Model file for the job. Use its own axes, mm. A direction names the side the tool comes from. Round coordinates to 2 decimals unless told otherwise and drop trailing zeros. Write each loop counter-clockwise with the first axis right and the second up, starting at its lowest first coordinate (ties: lowest second). Pieces come first, ordered by that corner, then holes. Notation, with made-up numbers: (-7.75, 89) - (42.25, 89) arc R9 ccw to (42.25, 100) - close; hole circle Ø6 at (-23.75, 42). An arc over 180 degrees is marked (long way). One line per item, written item: value.
Autodesk Inventor part; units mm, degrees
ref_plane "YZ Plane" through (0, 0, 0) normal (1, 0, 0) x (0, 1, 0)
ref_plane "XZ Plane" through (0, 0, 0) normal (0, 1, 0) x (-1, 0, 0)
ref_plane "XY Plane" through (0, 0, 0) normal (0, 0, 1) x (1, 0, 0)
sketch "Sketch1" plane through (0, 0, 0) normal (0, 0, 1) x (1, 0, 0)
  line L0 (-43.5443, 19.427) -> (49.4557, 19.427)
  line L1 (52.4557, 16.427) -> (52.4557, -43.573)
  line L2 (49.4557, -46.573) -> (-43.5443, -46.573)
  line L3 (-46.5443, -43.573) -> (-46.5443, 16.427)
  arc A0 (-43.5443, 19.427) -> (-46.5443, 16.427) centre (-43.5443, 16.427) ccw
  arc A1 (-46.5443, -43.573) -> (-43.5443, -46.573) centre (-43.5443, -43.573) ccw
  arc A2 (49.4557, -46.573) -> (52.4557, -43.573) centre (49.4557, -43.573) ccw
  arc A3 (52.4557, 16.427) -> (49.4557, 19.427) centre (49.4557, 16.427) ccw
  point P0 (0, 0)
  point P1 (0, 0)
  point P2 (-46.5443, 19.427)
  point P3 (52.4557, -46.573)
  point P4 (52.4557, 19.427)
  dimension "d0" = 99
  dimension "d1" = 66
  dimension "d2" = 3
extrude "Extrusion1" add sketch "Sketch1" along normal blind 1.27
sketch "Sketch2" plane through (0, 0, 1.27) normal (0, 0, 1) x (1, 0, 0)
  line L0 (-46.5443, 16.427) -> (-46.5443, -43.573)
  line L1 (49.4557, 19.427) -> (-43.5443, 19.427)
  circle A0 centre (-42.7343, 15.617) radius 1.5875
  line L2 (-50.0562, -13.573) -> (79.0191, -13.573) construction
  line L3 (2.9557, 30.2203) -> (2.9557, -48.7988) construction
  circle A1 centre (-42.7343, -42.763) radius 1.5875
  circle A2 centre (48.6457, 15.617) radius 1.5875
  circle A3 centre (48.6457, -42.763) radius 1.5875
  point P0 (0, 0)
  dimension "d8" = 3.175
  dimension "d9" = 3.81
  dimension "d10" = 3.81
extrude "Extrusion2" cut sketch "Sketch2" against normal blind 25.4
sketch "Sketch3" plane through (0, 0, 1.27) normal (0, 0, 1) x (1, 0, 0)
  circle A0 centre (48.6457, 15.617) radius 1.5875
  circle A1 centre (-42.7343, 15.617) radius 1.5875
  circle A2 centre (-42.7343, -42.763) radius 1.5875
  circle A3 centre (48.6457, -42.763) radius 1.5875
  line L0 (49.4557, 19.427) -> (-43.5443, 19.427)
  arc A4 (-43.5443, 19.427) -> (-46.5443, 16.427) centre (-43.5443, 16.427) ccw
  line L1 (-46.5443, 16.427) -> (-46.5443, -43.573) construction
  arc A5 (-46.5443, -43.573) -> (-43.5443, -46.573) centre (-43.5443, -43.573) ccw
  line L2 (-43.5443, -46.573) -> (49.4557, -46.573)
  arc A6 (49.4557, -46.573) -> (52.4557, -43.573) centre (49.4557, -43.573) ccw
  line L3 (52.4557, -43.573) -> (52.4557, 16.427)
  arc A7 (52.4557, 16.427) -> (49.4557, 19.427) centre (49.4557, 16.427) ccw
  arc A8 (-43.5443, 19.427) -> (-46.5443, 16.427) centre (-43.5443, 16.427) ccw
  line L4 (49.4557, 19.427) -> (-43.5443, 19.427)
  circle A9 centre (48.6457, 15.617) radius 1.5875
  circle A10 centre (-42.7343, 15.617) radius 1.5875
  circle A11 centre (-42.7343, -42.763) radius 1.5875
  circle A12 centre (48.6457, -42.763) radius 1.5875
  arc A13 (52.4557, 16.427) -> (49.4557, 19.427) centre (49.4557, 16.427) ccw
  line L5 (52.4557, 16.427) -> (52.4557, -43.573)
  arc A14 (49.4557, -46.573) -> (52.4557, -43.573) centre (49.4557, -43.573) ccw
  line L6 (49.4557, -46.573) -> (-43.5443, -46.573)
  arc A15 (-46.5443, -43.573) -> (-43.5443, -46.573) centre (-43.5443, -43.573) ccw
  line L7 (-46.5443, -43.573) -> (-46.5443, 16.427)
  arc A16 (-43.5443, 19.427) -> (-46.5443, 16.427) centre (-43.5443, 16.427) ccw
  line L8 (-43.5443, 19.427) -> (49.4557, 19.427)
  line L9 (-43.5443, 19.427) -> (49.4557, 19.427)
  line L10 (-40.8039, 19.427) -> (-40.8039, -46.573) construction
  line L11 (49.4557, -46.573) -> (-43.5443, -46.573)
  line L12 (-40.8039, 19.427) -> (-51.3078, 19.427) construction
  line L13 (-40.8039, -46.573) -> (-51.3078, -46.573) construction
  line L14 (-40.8039, -21.173) -> (-51.3078, -21.173) construction
  line L15 (-40.8039, -5.973) -> (-51.3078, -5.973) construction
  line L16 (-46.5443, -43.573) -> (-46.5443, 16.427)
  line L17 (-46.5443, -5.973) -> (-40.8039, -5.973)
  line L18 (-40.8039, -5.973) -> (-40.8039, -21.173)
  line L19 (-40.8039, -21.173) -> (-46.5443, -21.173)
  line L20 (-46.5443, -21.173) -> (-46.5443, -5.973)
  point P0 (0, 0)
  dimension "d13" = 25.4
  dimension "d14" = 25.4
  dimension "d15" = 5.7404
extrude "Extrusion3" cut sketch "Sketch3" against normal blind 25.4 contours L17 L18 L19 L7
fillet "Fillet1" radius 3.175 2 edges at (-46.5443, -21.173, 0.635) (-46.5443, -5.973, 0.635)
sketch "Sketch9" plane through (0, 0, 1.27) normal (0, 0, 1) x (1, 0, 0)
  arc A0 (-43.5443, 19.427) -> (-46.5443, 16.427) centre (-43.5443, 16.427) ccw
  line L0 (-46.5443, -2.798) -> (-46.5443, 16.427) construction
  line L1 (-46.5443, 16.427) -> (-46.5443, -2.798)
  line L2 (-43.5443, 19.427) -> (-26.5771, 19.427) construction
  line L3 (49.4557, 19.427) -> (-43.5443, 19.427)
  line L4 (-45.6657, 18.5483) -> (-26.5771, -0.5403) construction
  line L5 (-45.6657, 18.5483) -> (-18.6704, 18.5483) construction
  circle A1 centre (-45.6657, 18.5483) radius 7.1603
  arc A2 (-46.5443, -2.798) -> (-43.3693, -5.973) centre (-43.3693, -2.798) ccw
  line L6 (-43.3693, -5.973) -> (-40.8039, -5.973)
  line L7 (-40.8039, -5.973) -> (-40.8039, -21.173)
  line L8 (-40.8039, -21.173) -> (-43.3693, -21.173)
  arc A3 (-43.3693, -21.173) -> (-46.5443, -24.348) centre (-43.3693, -24.348) ccw
  line L9 (-46.5443, -24.348) -> (-46.5443, -43.573)
  arc A4 (-46.5443, -43.573) -> (-43.5443, -46.573) centre (-43.5443, -43.573) ccw
  line L10 (-43.5443, -46.573) -> (49.4557, -46.573)
  arc A5 (49.4557, -46.573) -> (52.4557, -43.573) centre (49.4557, -43.573) ccw
  line L11 (52.4557, -43.573) -> (52.4557, 16.427)
  arc A6 (52.4557, 16.427) -> (49.4557, 19.427) centre (49.4557, 16.427) ccw
  line L12 (49.4557, 19.427) -> (-43.5443, 19.427)
  arc A7 (-43.5443, 19.427) -> (-46.5443, 16.427) centre (-43.5443, 16.427) ccw
  line L13 (-46.5443, 16.427) -> (-46.5443, -2.798)
  circle A8 centre (48.6457, 15.617) radius 1.5875
  circle A9 centre (-42.7343, 15.617) radius 1.5875
  circle A10 centre (-42.7343, -42.763) radius 1.5875
  circle A11 centre (48.6457, -42.763) radius 1.5875
  line L14 (-75.7777, -13.573) -> (114.1059, -13.573) construction
  line L15 (2.9557, 31.1348) -> (2.9557, -53.319) construction
  circle A12 centre (-45.6657, -45.6944) radius 7.1603
  line L16 (2.9557, -58.2809) -> (2.9557, 26.1729) construction
  circle A13 centre (51.577, 18.5483) radius 7.1603
  circle A14 centre (51.577, -45.6944) radius 7.1603
  point P0 (0, 0)
  dimension "d28" = 45
extrude "Extrusion5" cut sketch "Sketch9" against normal blind 12.7 contours L3 A1 L1 A0 | A0 L1 A1 L3 | A13 L11 A6 L3 | L3 A6 L11 A13 | A14 L10 A5 L11 | L11 A5 L10 A14 | A12 L9 A4 L10 | L10 A4 L9 A12
sketch "Sketch10" plane through (0, 0, 1.27) normal (0, 0, 1) x (1, 0, 0)
  arc A0 (52.4557, -38.5882) -> (44.4708, -46.573) centre (51.577, -45.6944) ccw
  line L0 (52.4557, -38.5882) -> (52.4557, 11.4421)
  arc A1 (44.4708, 19.427) -> (52.4557, 11.4421) centre (51.577, 18.5483) ccw
  line L1 (44.4708, 19.427) -> (-38.5595, 19.427)
  arc A2 (-46.5443, 11.4421) -> (-38.5595, 19.427) centre (-45.6657, 18.5483) ccw
  line L2 (-46.5443, 11.4421) -> (-46.5443, -2.798)
  arc A3 (-46.5443, -2.798) -> (-43.3693, -5.973) centre (-43.3693, -2.798) ccw
  line L3 (-43.3693, -5.973) -> (-40.8039, -5.973)
  line L4 (-40.8039, -5.973) -> (-40.8039, -21.173)
  line L5 (-40.8039, -21.173) -> (-43.3693, -21.173)
  arc A4 (-43.3693, -21.173) -> (-46.5443, -24.348) centre (-43.3693, -24.348) ccw
  line L6 (-46.5443, -24.348) -> (-46.5443, -38.5882)
  arc A5 (-38.5595, -46.573) -> (-46.5443, -38.5882) centre (-45.6657, -45.6944) ccw
  line L7 (-38.5595, -46.573) -> (44.4708, -46.573)
  line L8 (-36.7645, -45.303) -> (43.1467, -45.303)
  line L9 (-36.7645, 18.157) -> (43.1467, 18.157)
  line L10 (44.4708, 19.427) -> (-38.5595, 19.427)
  line L11 (-36.7645, -45.303) -> (-37.2353, -45.303)
  arc A6 (-38.5595, -46.573) -> (-46.5443, -38.5882) centre (-45.6657, -45.6944) ccw
  line L12 (-36.7645, 18.157) -> (-37.2353, 18.157)
  line L13 (51.1857, 10.118) -> (51.1857, -37.264)
  arc A7 (44.4708, 19.427) -> (52.4557, 11.4421) centre (51.577, 18.5483) ccw
  line L14 (-39.5339, -5.973) -> (-39.5339, -21.173)
  line L15 (-45.2743, -2.798) -> (-39.5339, -5.973)
  line L16 (-39.5339, -21.173) -> (-45.2743, -24.348)
  line L17 (51.1857, 10.118) -> (52.4557, 10.118) construction
  line L18 (52.4557, -38.5882) -> (52.4557, 11.4421)
  line L19 (43.1467, 18.157) -> (43.1467, 19.427) construction
  arc A8 (43.1467, 18.157) -> (51.1857, 10.118) centre (51.577, 18.5483) ccw
  line L20 (-56.5649, -13.573) -> (80.9191, -13.573) construction
  line L21 (2.9557, 34.2968) -> (2.9557, -68.6615) construction
  arc A9 (51.1857, -37.264) -> (43.1467, -45.303) centre (51.577, -45.6944) ccw
  arc A10 (-45.2743, 10.118) -> (-37.2353, 18.157) centre (-45.6657, 18.5483) ccw
  arc A11 (-37.2353, -45.303) -> (-45.2743, -37.264) centre (-45.6657, -45.6944) ccw
  line L22 (-45.2743, 10.118) -> (-45.2743, -2.798)
  line L23 (-45.2743, -37.264) -> (-45.2743, -24.348)
  line L24 (-46.5443, -43.573) -> (-46.5443, -24.348)
  point P0 (0, 0)
  dimension "d31" = 1.27
  dimension "d32" = 1.27
  dimension "d35" = 1.27
  dimension "d36" = 1.27
  dimension "d39" = 3.175
  dimension "d40" = 3.175
  dimension "d42" = 1.27
  dimension "d43" = 1.27
  dimension "d44" = 1.2791
extrude "Extrusion6" cut sketch "Sketch10" against normal blind 7.62 contours L11 A11 L23 L16 L14 L15 L22 A10 L12 L9 A8 L13 A9 L8
sketch "Sketch13" plane through (0, 0, 1.27) normal (0, 0, 1) x (1, 0, 0)
  arc A0 (51.1857, -37.264) -> (43.1467, -45.303) centre (51.577, -45.6944) ccw
  line L0 (43.1467, -45.303) -> (-37.2353, -45.303)
  arc A1 (-37.2353, -45.303) -> (-45.2743, -37.264) centre (-45.6657, -45.6944) ccw
  line L1 (-45.2743, -37.264) -> (-45.2743, -24.348)
  line L2 (-45.2743, -24.348) -> (-39.5339, -21.173)
  line L3 (-39.5339, -21.173) -> (-39.5339, -5.973)
  line L4 (-39.5339, -5.973) -> (-45.2743, -2.798)
  line L5 (-45.2743, -2.798) -> (-45.2743, 10.118)
  arc A2 (-45.2743, 10.118) -> (-37.2353, 18.157) centre (-45.6657, 18.5483) ccw
  line L6 (-37.2353, 18.157) -> (43.1467, 18.157)
  arc A3 (43.1467, 18.157) -> (51.1857, 10.118) centre (51.577, 18.5483) ccw
  line L7 (51.1857, 10.118) -> (51.1857, -37.264)
  arc A4 (52.4557, -38.5882) -> (44.4708, -46.573) centre (51.577, -45.6944) ccw
  line L8 (52.4557, -38.5882) -> (52.4557, 11.4421)
  arc A5 (44.4708, 19.427) -> (52.4557, 11.4421) centre (51.577, 18.5483) ccw
  line L9 (44.4708, 19.427) -> (-38.5595, 19.427)
  arc A6 (-46.5443, 11.4421) -> (-38.5595, 19.427) centre (-45.6657, 18.5483) ccw
  line L10 (-46.5443, 11.4421) -> (-46.5443, -2.798)
  arc A7 (-46.5443, -2.798) -> (-43.3693, -5.973) centre (-43.3693, -2.798) ccw
  line L11 (-43.3693, -5.973) -> (-40.8039, -5.973)
  line L12 (-40.8039, -5.973) -> (-40.8039, -21.173)
  line L13 (-40.8039, -21.173) -> (-43.3693, -21.173)
  arc A8 (-43.3693, -21.173) -> (-46.5443, -24.348) centre (-43.3693, -24.348) ccw
  line L14 (-46.5443, -24.348) -> (-46.5443, -38.5882)
  arc A9 (-38.5595, -46.573) -> (-46.5443, -38.5882) centre (-45.6657, -45.6944) ccw
  line L15 (-38.5595, -46.573) -> (44.4708, -46.573)
  point P0 (0, 0)
extrude "Extrusion9" add sketch "Sketch13" along normal blind 1.27 and the other way blind 1.27 contours A0 L0 A1 L1 L2 L3 L4 L5 A2 L6 A3 L7
properties part number "battbase__lid_final"
1. Tool access for faces 4 (the face through (-45.64, -22.13, 0.63)), 5 (the face through (45.548, -39.789, 1.896)), 6 (the face through (-42.36, -4.41, 1.9)): list every direction of +Z, -Z, +X, -X, +Y, -Y with a clear straight run to the whole face (end or side of a thin tool).
Report:
face 4: +Z, -Z, -X
face 5: +Z, +X, -Y
face 6: +Z, -X
2. Band-saw the part on A-A on y = -19.5. Write the cut outline in (x, z), plus the area to 3 significant figures.
Report:
outline: (-40.8, 0) - (52.46, 0) - (52.46, 1.27) - (51.19, 1.27) - (51.19, 2.54) - (-39.53, 2.54) - (-39.53, 1.27) - (-40.8, 1.27) - close
area: 234 mm²
3. Wall check: probe 1 along X at (y, z) = (-16, 0.75); probe 2 along Y at (x, z) = (5, 1.35); probe 3 along X at (y, z) = (-8, 2.45). Give the ranges that are in metal, low to high. Write a range as [from, to].
Report:
probe 1: [-40.8, 52.46]
probe 2: [-45.3, 18.16]
probe 3: [-39.53, 51.19]
4. Band-saw the part on C-C on x = 5. Write the cut outline in (y, z), plus the area to 3 significant figures.
Report:
outline: (-46.57, 0) - (19.43, 0) - (19.43, 1.27) - (18.16, 1.27) - (18.16, 2.54) - (-45.3, 2.54) - (-45.3, 1.27) - (-46.57, 1.27) - close
area: 164 mm²
5. Mould opens along Y. For faces 1 (the face through (-39.76, -39.665, 1.896)), 2 (the face through (2, -13, 2.54)), 3 (the face through (-45.59, -5.068, 0.626)) say: released by +Y, released by -Y, zero draft, split by the parting line, or undercut.
Report:
face 1: released by -Y
face 2: zero draft
face 3: undercut
6. Drop flat-ended pins along their axis: pin 1 (1 mm diameter, centred on y = -10.5, z = 1, fed in from -X); pin 2 (1 mm diameter, centred on x = -42, z = 0.5, fed in from -Y); pin 3 (1 mm diameter, centred on y = -20, z = 2, fed in from +X). Give the stop position or say it passes through.
Report:
pin 1: x = -40.8
pin 2: y = -39.87
pin 3: x = 51.19
